Read the model definition and answer for the solid it produces. Units are mm, in the model's axes. Give positions to 0.01 mm unless a question says otherwise; leave off trailing zeros. Order: outer loops, then holes, each group sorted by start corner. A loop starts at its lowest first (then second) coordinate and runs counter-clockwise, first axis right, second up. Notation, with made-up numbers: (-12, 74.5) - (5, 74.5) arc R6 ccw to (5, 82.5) - close; hole circle Ø5 at (-7.75, 4.25). An arc over 180 degrees is marked (long way). Use a Markdown table: item, result. Add a question column.
1. A cutting plane is placed at B-B on x = -0.85. Determine the outline of the cut face in (y, z) (1 decimal), and give its area (3 significant figures).
2. Consider L1, parallel to Y at x = 0.2, z = -11; L2, parallel to Z at x = 1.4, y = 0.5; L3, parallel to Z at x = -0.6, y = -1.25. Determine where each line is inside the solid, lowest interval first.
3. A cutting plane is placed at A-A on z = -11. Determine the outline of the cut face in (x, y), and give its area (3 significant figures).
4. For a pull along Z with two mould halves and no side action, classify faces 1 (the flat face through (0, -3.81, 0)), 2 (the cylindrical face through (-0.022, 0.07, 9.414)), 3 (the flat face through (0, 0, 15.24)) as released by +Z, released by -Z, zero draft, split by the parting line, or undercut.
5. A cutting plane is placed at C-C on y = -0.5. Determine the outline of the cut face in (x, z).
```python
from build123d import *

# Parameters (mm, degrees)
SKETCH1_W           = 3.175
SKETCH1_H           = 7.62
BOSS_EXTRUDE1_DEPTH = 15.24
SKETCH3_R           = 1.5875
CUT_EXTRUDE2_DEPTH  = 4.175
SKETCH5_R           = 1.5875
CUT_EXTRUDE4_DEPTH  = 4.175


with BuildPart() as part:
    # Sketch1 → Boss-Extrude1 (new body)
    with BuildSketch(Plane.XY):
        Rectangle(SKETCH1_W, SKETCH1_H)
    boss_extrude1 = extrude(amount=BOSS_EXTRUDE1_DEPTH)

    # Mirror1: Boss-Extrude1 across plane
    add(boss_extrude1.mirror(Plane.XY))

    # Sketch3 → Cut-Extrude2 (cut, through all)
    with BuildSketch(Plane.ZY.offset(1.5875)):
        with Locations((-3.175, 0)):
            Circle(SKETCH3_R)
        with Locations((3.175, 0)):
            Circle(SKETCH3_R)
    extrude(amount=-CUT_EXTRUDE2_DEPTH, mode=Mode.SUBTRACT)

    # Sketch5 → Cut-Extrude4 (cut, through all)
    with BuildSketch(Plane.ZY.offset(1.5875)):
        with Locations((-11, 0)):
            Circle(SKETCH5_R)
        with Locations((11, 0)):
            Circle(SKETCH5_R)
    extrude(amount=-CUT_EXTRUDE4_DEPTH, mode=Mode.SUBTRACT)


solid = part.part
```
Output values:
| question | item | result |
|---|---|---|
| 1 | outline | (-3.8, -15.2) - (3.8, -15.2) - (3.8, 15.2) - (-3.8, 15.2) - close; hole circle Ø3.2 at (0, -11); hole circle Ø3.2 at (0, -3.2); hole circle Ø3.2 at (0, 3.2); hole circle Ø3.2 at (0, 11) |
| 1 | area | 201 mm² |
| 2 | L1 | -3.81 to -1.59, 1.59 to 3.81 |
| 2 | L2 | -15.24 to -12.51, -9.49 to -4.68, -1.67 to 1.67, 4.68 to 9.49, 12.51 to 15.24 |
| 2 | L3 | -15.24 to -11.98, -10.02 to -4.15, -2.2 to 2.2, 4.15 to 10.02, 11.98 to 15.24 |
| 3 | outline | (-1.59, -3.81) - (1.59, -3.81) - (1.59, -1.59) - (-1.59, -1.59) - close; (-1.59, 1.59) - (1.59, 1.59) - (1.59, 3.81) - (-1.59, 3.81) - close |
| 3 | area | 14.1 mm² |
| 4 | face 1 | zero draft |
| 4 | face 2 | undercut |
| 4 | face 3 | released by +Z |
| 5 | outline | (-1.59, -15.24) - (1.59, -15.24) - (1.59, -12.51) - (-1.59, -12.51) - close; (-1.59, -9.49) - (1.59, -9.49) - (1.59, -4.68) - (-1.59, -4.68) - close; (-1.59, -1.67) - (1.59, -1.67) - (1.59, 1.67) - (-1.59, 1.67) - close; (-1.59, 4.68) - (1.59, 4.68) - (1.59, 9.49) - (-1.59, 9.49) - close; (-1.59, 12.51) - (1.59, 12.51) - (1.59, 15.24) - (-1.59, 15.24) - close |
